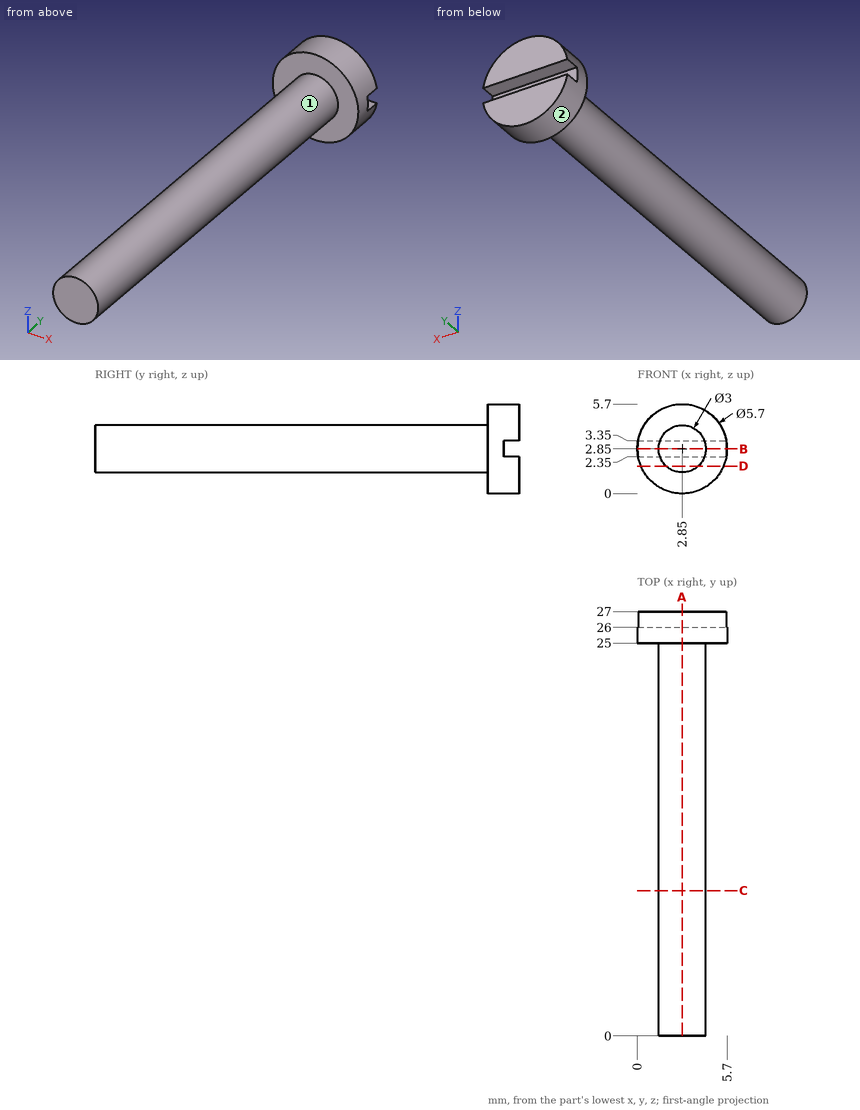
Answer from the drawing. Dimensions are ordinates in mm from the lowest x, y and z of the part. A direction names the side the tool comes from. Give positions to 0.01 mm unless a question says otherwise; leave off trailing zeros. Write each loop counter-clockwise with the first axis right and the second up, starting at its lowest first coordinate (ties: lowest second). Pieces come first, ordered by that corner, then holes.
1) Section A-A (x = 2.85) is taken. Write down the section's boundary in (y, z).
2) Given P1, Ø2, axis at y = 22.5, z = 3, coming from the +X side; P2, Ø1.1, axis at x = 2, y = 26.5, coming from the -Z side; P3, Ø0.5, axis at x = 3.5, z = 3, coming from the +Y side, each flat-ended and moving along its own axis, determine where each tip first touches the part or whether it passes through.
3) A tool of negligible diameter and unlimited length cuts with its end or side. For the marked faces 1 and 2, from which of +Z, -Z, +X, -X, +Y, -Y can it reach the whole face along a straight path? Write none if from no direction.
4) Section C-C (y = 9.25) is taken. Write down the section's boundary in (x, z), and give its area (3 significant figures).
5) Find the intervals of material crossed by L1, parallel to Y at x = 2.1, z = 3.05; L2, parallel to Z at x = 2.75, y = 21.25; L3, parallel to Y at x = 4.15, z = 3.85, in increasing order.
6) Section B-B (z = 2.85) is taken. Write down the section's boundary in (x, y), and give its area (3 significant figures).
7) Section D-D (z = 1.75) is taken. Write down the section's boundary in (x, y).
Response:
1. outline: (0, 1.35) - (25, 1.35) - (25, 0) - (27, 0) - (27, 2.35) - (26, 2.35) - (26, 3.35) - (27, 3.35) - (27, 5.7) - (25, 5.7) - (25, 4.35) - (0, 4.35) - close
2. P1: stops at x = 4.35
2. P2: stops at z = 0.02
2. P3: stops at y = 26
3. face 1: -Y
3. face 2: +Y, -Y
4. outline: circle Ø3 at (2.85, 2.85)
4. area: 7.07 mm2
5. L1: y = 0 to 26
5. L2: z = 1.35 to 4.35
5. L3: y = 25 to 27
6. outline: (0, 25) - (1.35, 25) - (1.35, 0) - (4.35, 0) - (4.35, 25) - (5.7, 25) - (5.7, 26) - (0, 26) - close
6. area: 80.7 mm2
7. outline: (0.22, 25) - (1.83, 25) - (1.83, 0) - (3.87, 0) - (3.87, 25) - (5.48, 25) - (5.48, 27) - (0.22, 27) - close
